Geometry: final body of the model. Coordinates: model frame, mm. Face numbers are marked on the shaded views. A direction names the side the tool comes from. Coordinates: 2 decimals unless noted, no trailing zeros. Write each loop counter-clockwise with the first axis right and the second up, starting at its lowest first coordinate (ties: lowest second). Pieces come first, ordered by that corner, then holes. Notation, with made-up numbers: (-32, -32) - (-9, -32) arc R23 ccw to (-9, -23) - close; hole circle Ø7 at (66, 18). An arc over 180 degrees is marked (long way). Put each result on its own line as item: value.
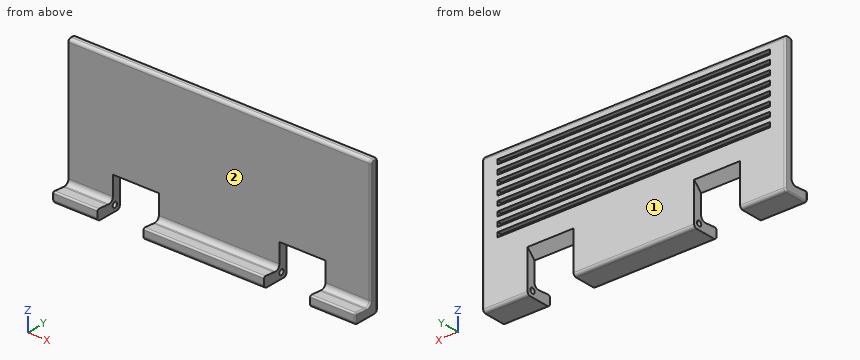
```python
from build123d import *

# Parameters (mm, degrees)
F1_DEPTH      = 100
F1_DEPTH_BACK = 100
F2_R          = 1
F5_DEPTH      = 70.2
F5_DEPTH_BACK = 70.2
F6_DEPTH      = 39.8
F6_DEPTH_BACK = 39.8
F3_R          = 1.7
F7_DEPTH      = 200.001
F9_DEPTH      = 90
F9_DEPTH_BACK = 90
F10_R         = 1.7
F11_DEPTH     = 20
F12_R         = 2.1690040251
F13_DEPTH     = 20


with BuildPart() as f1:
    # F0 (on Right) → F1 (new body, two sides)
    with BuildSketch(Plane.YZ) as f1_sk:
        with BuildLine():
            Line((0, 2), (0, 88))
            ThreePointArc((0, 88), (-0.5857864376, 89.4142135624), (-2, 90))
            Line((-2, 90), (-3.5, 90))
            ThreePointArc((-3.5, 90), (-4.9142135624, 89.4142135624), (-5.5, 88))
            Line((-5.5, 88), (-5.5, 43.945170586))
            Line((-5.5, 43.945170586), (-5.5, 9.2603986447))
            ThreePointArc((-5.5, 9.2603986447), (-6.468671533, 7.0527517845), (-8.7491364396, 6.27076137))
            Line((-8.7491364396, 6.27076137), (-9.8321819194, 6.36101516))
            Line((-9.8321819194, 6.36101516), (-16.4169545201, 6.90974621))
            ThreePointArc((-16.4169545201, 6.90974621), (-17.177109489, 6.6490827385), (-17.5, 5.9132004518))
            Line((-17.5, 5.9132004518), (-17.5, 2))
            ThreePointArc((-17.5, 2), (-16.9142135624, 0.5857864376), (-15.5, 0))
            Line((-15.5, 0), (-2, 0))
            ThreePointArc((-2, 0), (-0.5857864376, 0.5857864376), (0, 2))
        make_face()
    extrude(amount=F1_DEPTH)
    extrude(f1_sk.sketch, amount=-F1_DEPTH_BACK)

    # F2
    f2_edges = [f1.edges().sort_by_distance(p)[0] for p in [
        (-100, 0, 45),
        (100, 0, 45),
    ]]
    fillet(f2_edges, radius=F2_R)

    # F4 (on Right) → F5 (cut, two sides)
    with BuildSketch(Plane.YZ) as f5_sk:
        Polygon((-8.8815924794, 6.6997300052), (-19.3425188781, 7.6679212159), (-19.3425188781, 0), (0, 0), (0, 27.5), (-5.5, 22), (-5.5, 9.4664877642), align=None)
    extrude(amount=F5_DEPTH, mode=Mode.SUBTRACT)
    extrude(f5_sk.sketch, amount=-F5_DEPTH_BACK, mode=Mode.SUBTRACT)

    # F0 (on Right) → F6 (join, two sides)
    with BuildSketch(Plane.YZ) as f6_sk:
        with BuildLine():
            Line((0, 2), (0, 88))
            ThreePointArc((0, 88), (-0.5857864376, 89.4142135624), (-2, 90))
            Line((-2, 90), (-3.5, 90))
            ThreePointArc((-3.5, 90), (-4.9142135624, 89.4142135624), (-5.5, 88))
            Line((-5.5, 88), (-5.5, 43.945170586))
            Line((-5.5, 43.945170586), (-5.5, 9.2603986447))
            ThreePointArc((-5.5, 9.2603986447), (-6.468671533, 7.0527517845), (-8.7491364396, 6.27076137))
            Line((-8.7491364396, 6.27076137), (-9.8321819194, 6.36101516))
            Line((-9.8321819194, 6.36101516), (-16.4169545201, 6.90974621))
            ThreePointArc((-16.4169545201, 6.90974621), (-17.177109489, 6.6490827385), (-17.5, 5.9132004518))
            Line((-17.5, 5.9132004518), (-17.5, 2))
            ThreePointArc((-17.5, 2), (-16.9142135624, 0.5857864376), (-15.5, 0))
            Line((-15.5, 0), (-2, 0))
            ThreePointArc((-2, 0), (-0.5857864376, 0.5857864376), (0, 2))
        make_face()
    extrude(amount=F6_DEPTH)
    extrude(f6_sk.sketch, amount=-F6_DEPTH_BACK)

    # F3 (on face) → F7 (cut, through all)
    with BuildSketch(Plane.YZ.offset(100)):
        with Locations((-3.9070966475, 3.9112776819)):
            Circle(F3_R)
    extrude(amount=-F7_DEPTH, mode=Mode.SUBTRACT)

    # F8 (on Right) → F9 (cut, two sides)
    with BuildSketch(Plane.YZ) as f9_sk:
        Polygon((1.8498107092, 85), (0, 85), (-3, 85), (0, 82), (0, 79), (-3, 79), (0, 76), (0, 73), (-3, 73), (0, 70), (0, 67), (-3, 67), (0, 64), (0, 61), (-3, 61), (0, 58), (0, 55), (-3, 55), (0, 52), (0, 49), (-3, 49), (0, 46), (0, 43), (-3, 43), (0, 40), (1.8498107092, 39.9083867669), align=None)
    extrude(amount=-F9_DEPTH, mode=Mode.SUBTRACT)
    extrude(f9_sk.sketch, amount=F9_DEPTH_BACK, mode=Mode.SUBTRACT)

    # F10 (on face) → F11 (join)
    with BuildSketch(Plane.YZ.offset(100)):
        with Locations((-3.9070966475, 3.9112776819)):
            Circle(F10_R)
    extrude(amount=-F11_DEPTH)

    # F12 (on face) → F13 (join)
    with BuildSketch(Plane(origin=(-100, 0, 0), x_dir=(0, -1, 0), z_dir=(-1, 0, 0))):
        with Locations((3.9070966475, 3.9112776819)):
            Circle(F12_R)
    extrude(amount=-F13_DEPTH)


solid = f1.part
```
1. Section query C-C (y = -13.5). Count the separate pieces of the cut face and the enclosed holes in it, then the cut area to 3 significant figures.
Answer below:
separate pieces: 3
enclosed holes: 0
area: 927 mm²
2. Set-up query: the marked faces 1 and 2. Return all of +Z, -Z, +X, -X, +Y, -Y with unobstructed straight access to the full face (end or side cutting, diameter ignored); none if empty.
Answer below:
face 1: +Z, -Z, +X, -X, +Y
face 2: +Z, +X, -X, -Y
3. Section query A-A (z = 36). Return loops of the section in (x, y), then the cut area to 3 significant figures.
Answer below:
outline: (-100, -4.5) arc R1 ccw to (-99, -5.5) - (99, -5.5) arc R1 ccw to (100, -4.5) - (100, -1) arc R1 ccw to (99, 0) - (-99, 0) arc R1 ccw to (-100, -1) - close
area: 1,100 mm²
4. Pin query (flat end, axial travel): pin 1 Ø6 at (x, y) = (-54.5, -5) entering from -Z; pin 2 Ø3 at (x, z) = (-41, 31) entering from -Y; pin 3 Ø2 at (x, z) = (-25, 47.5) entering from +Y. Return the tip coordinate at first contact, or that it passes through.
Answer below:
pin 1: stops at z = 22
pin 2: stops at y = -5.5
pin 3: stops at y = -0.5
5. Ray query, probe 1 along X at (y, z) = (-3.25, 20.5); probe 2 along X at (y, z) = (-3.75, 5); probe 3 along Y at (x, z) = (35.5, 9). Return the intervals inside material, ascending. Write a range as from..to.
Answer below:
probe 1: x = -100..-70.2, -39.8..39.8, 70.2..100
probe 2: x = -100..-80, 80..100
probe 3: y = -5.51..0
